Build history of the part. All positions in model axes, mm. Face numbers are marked on the shaded views. Give positions to 0.01 mm unless a question says otherwise; leave off trailing zeros. Write each loop counter-clockwise with the first axis right and the second up, starting at its lowest first coordinate (ties: lowest second). Pieces come first, ordered by that corner, then holes.
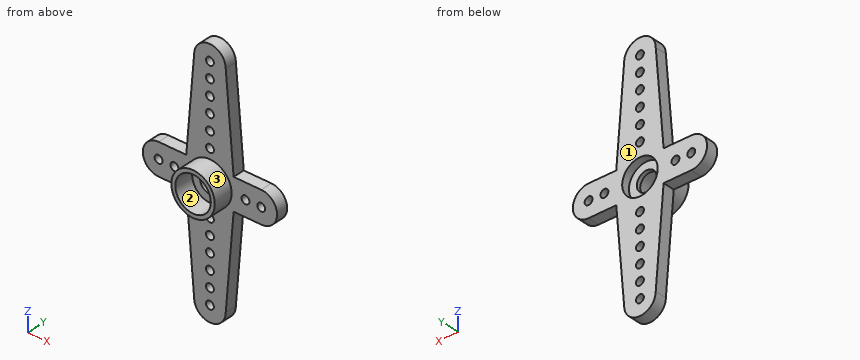
from build123d import *

# Parameters (mm, degrees)
ESQUISSE1_R             = 2.75
ESQUISSE1_R_2           = 2.25
BOSS_EXTRU_1_DEPTH      = 2.5
BOSS_EXTRU_2_DEPTH      = 1.5
ESQUISSE4_R             = 2.25
ENL_V_MAT_EXTRU_1_DEPTH = 1
ENL_V_MAT_EXTRU_2_REACH = 5
ESQUISSE5_R             = 1.25
ESQUISSE6_R             = 0.5
ENL_V_MAT_EXTRU_3_DEPTH = 5


with BuildPart() as part:
    # Esquisse1 → Boss.-Extru.1 (new body)
    with BuildSketch(Plane(origin=(0, 0, 0), x_dir=(1, 0, 0), z_dir=(0, 1, 0))):
        Circle(ESQUISSE1_R)
        Circle(ESQUISSE1_R_2, mode=Mode.SUBTRACT)
    extrude(amount=BOSS_EXTRU_1_DEPTH)

    # Esquisse3 → Boss.-Extru.2 (add)
    with BuildSketch(Plane(origin=(0, 2.5, 0), x_dir=(1, 0, 0), z_dir=(0, 1, 0))):
        with BuildLine():
            Line((-6.5, 2), (-3, 2))
            Line((-3, 2), (-2, 14))
            ThreePointArc((-2, 14), (0, 16), (2, 14))
            Line((2, 14), (3, 2))
            Line((3, 2), (6.5, 2))
            ThreePointArc((6.5, 2), (8.5, 0), (6.5, -2))
            Line((6.5, -2), (3, -2))
            Line((3, -2), (2, -14))
            ThreePointArc((2, -14), (0, -16), (-2, -14))
            Line((-2, -14), (-3, -2))
            Line((-3, -2), (-6.5, -2))
            ThreePointArc((-6.5, -2), (-8.5, 0), (-6.5, 2))
        make_face()
    extrude(amount=BOSS_EXTRU_2_DEPTH)

    # Esquisse4 → Enlèv. mat.-Extru.1 (cut)
    with BuildSketch(Plane(origin=(0, 4, 0), x_dir=(1, 0, 0), z_dir=(0, 1, 0))):
        Circle(ESQUISSE4_R)
    extrude(amount=-ENL_V_MAT_EXTRU_1_DEPTH, mode=Mode.SUBTRACT)

    # Esquisse5 → Enlèv. mat.-Extru.2 (cut, up to next)
    with BuildSketch(Plane(origin=(0, 3, 0), x_dir=(1, 0, 0), z_dir=(0, 1, 0)), mode=Mode.PRIVATE) as enl_v_mat_extru_2_sk1:
        Circle(ESQUISSE5_R)
    enl_v_mat_extru_2_tool1 = extrude(enl_v_mat_extru_2_sk1.sketch, amount=-ENL_V_MAT_EXTRU_2_REACH, mode=Mode.PRIVATE) & part.part
    add(enl_v_mat_extru_2_tool1.solids().sort_by_distance((0, 3, 0))[0], mode=Mode.SUBTRACT)

    # Esquisse6 → Enlèv. mat.-Extru.3 (cut, through all)
    with BuildSketch(Plane(origin=(0, 4, 0), x_dir=(1, 0, 0), z_dir=(0, 1, 0))):
        with Locations((4.5, 0)):
            Circle(ESQUISSE6_R)
        with Locations((6.5, 0)):
            Circle(ESQUISSE6_R)
        with Locations((-4.5, 0)):
            Circle(ESQUISSE6_R)
        with Locations((-6.5, 0)):
            Circle(ESQUISSE6_R)
        with Locations((0, 14)):
            Circle(ESQUISSE6_R)
        with Locations((0, 12)):
            Circle(ESQUISSE6_R)
        with Locations((0, 10)):
            Circle(ESQUISSE6_R)
        with Locations((0, 8)):
            Circle(ESQUISSE6_R)
        with Locations((0, 6)):
            Circle(ESQUISSE6_R)
        with Locations((0, 4)):
            Circle(ESQUISSE6_R)
        with Locations((0, -4)):
            Circle(ESQUISSE6_R)
        with Locations((0, -6)):
            Circle(ESQUISSE6_R)
        with Locations((0, -8)):
            Circle(ESQUISSE6_R)
        with Locations((0, -10)):
            Circle(ESQUISSE6_R)
        with Locations((0, -12)):
            Circle(ESQUISSE6_R)
        with Locations((0, -14)):
            Circle(ESQUISSE6_R)
    extrude(amount=-ENL_V_MAT_EXTRU_3_DEPTH, mode=Mode.SUBTRACT)


solid = part.part
(1) Saw through at A-A, the plane x = -4.5. List the corners of the cut face in (y, z).
(2) Probe line 1 (X direction, y = 2.7, z = 0); line 2 (Z direction, x = -6.5, y = 3.5); line 3 (Z direction, x = 0, y = 0.5). List the from-to ranges inside material, lowest first.
(3) Mould opens along Z. For the marked faces 1, 2 and 3 say: +Z half, -Z half, draft (parallel to the pull), parting line (faces both ways), or undercut.
(4) Saw through at B-B, the plane y = 3.5. Give the number of separate pieces and of enclosed holes in the cut face, plus the area to 3 significant figures.
(5) Saw through at C-C, the plane z = -4. List the corners of the cut face in (x, y).
(6) Drop flat-ended pins along their axis: pin 1 (0.8 mm diameter, centred on x = 5.5, y = 3.5, fed in from +Z); pin 2 (0.8 mm diameter, centred on x = -5.5, y = 3.5, fed in from -Z); pin 3 (4 mm diameter, centred on x = 0, z = 0, fed in from -Y); pin 4 (5 mm diameter, centred on x = 3, z = -7, fed in from +Y). Give the stop position or say it passes through.
Computed values:
1. outline: (2.5, -2) - (4, -2) - (4, -0.5) - (2.5, -0.5) - close; (2.5, 0.5) - (4, 0.5) - (4, 2) - (2.5, 2) - close
2. line 1: x = -8.5 to -7, -6 to -5, -4 to -1.25, 1.25 to 4, 5 to 6, 7 to 8.5
2. line 2: z = -2 to -0.5, 0.5 to 2
2. line 3: z = -2.75 to -2.25, 2.25 to 2.75
3. face 1: draft
3. face 2: undercut
3. face 3: parting line
4. separate pieces: 1
4. enclosed holes: 17
4. area: 169 mm2
5. outline: (-2.83, 2.5) - (-0.5, 2.5) - (-0.5, 4) - (-2.83, 4) - close; (0.5, 2.5) - (2.83, 2.5) - (2.83, 4) - (0.5, 4) - close
6. pin 1: stops at z = 2
6. pin 2: stops at z = -2
6. pin 3: stops at y = 2.5
6. pin 4: stops at y = 4
